```python
from build123d import *

# Parameters (mm, degrees)
SKETCH_1_R          = 1.65
EXTRUDE_1_DEPTH     = 20
CUT_EXTRUDE_START   = -15
SKETCH_4_R          = 1.65
CUT_EXTRUDE_1_DEPTH = 15
FILLET_1_R          = 10
FILLET_2_R          = 5


with BuildPart() as part:
    # ｽｹｯﾁ1 → ﾎﾞｽ - 押し出し1 (new body)
    with BuildSketch(Plane(origin=(0, 0, 0), x_dir=(1, 0, 0), z_dir=(0, 1, 0))):
        with BuildLine():
            Line((20.396078054, 5), (20.396078054, -5))
            ThreePointArc((20.396078054, -5), (19.876430019, -6.776985295), (19.202290705, -8.501295883))
            ThreePointArc((19.202290705, -8.501295883), (18.958497792, -12.709351685), (21.542725681, -16.039356915))
            ThreePointArc((21.542725681, -16.039356915), (22.273863607, -22.273863607), (16.039356915, -21.542725681))
            ThreePointArc((16.039356915, -21.542725681), (12.709351685, -18.958497792), (8.501295883, -19.202290705))
            ThreePointArc((8.501295883, -19.202290705), (6.776985295, -19.876430019), (5, -20.396078054))
            Line((5, -20.396078054), (-5, -20.396078054))
            ThreePointArc((-5, -20.396078054), (-6.776985295, -19.876430019), (-8.501295883, -19.202290705))
            ThreePointArc((-8.501295883, -19.202290705), (-12.709351685, -18.958497792), (-16.039356915, -21.542725681))
            ThreePointArc((-16.039356915, -21.542725681), (-22.273863607, -22.273863607), (-21.542725681, -16.039356915))
            ThreePointArc((-21.542725681, -16.039356915), (-18.958497792, -12.709351685), (-19.202290705, -8.501295883))
            ThreePointArc((-19.202290705, -8.501295883), (-19.876430019, -6.776985295), (-20.396078054, -5))
            Line((-20.396078054, -5), (-20.396078054, 5))
            ThreePointArc((-20.396078054, 5), (-19.876430019, 6.776985295), (-19.202290705, 8.501295883))
            ThreePointArc((-19.202290705, 8.501295883), (-18.958497792, 12.709351685), (-21.542725681, 16.039356915))
            ThreePointArc((-21.542725681, 16.039356915), (-22.273863607, 22.273863607), (-16.039356915, 21.542725681))
            ThreePointArc((-16.039356915, 21.542725681), (-12.709351685, 18.958497792), (-8.501295883, 19.202290705))
            ThreePointArc((-8.501295883, 19.202290705), (-6.776985295, 19.876430019), (-5, 20.396078054))
            Line((-5, 20.396078054), (5, 20.396078054))
            ThreePointArc((5, 20.396078054), (6.776985295, 19.876430019), (8.501295883, 19.202290705))
            ThreePointArc((8.501295883, 19.202290705), (12.709351685, 18.958497792), (16.039356915, 21.542725681))
            ThreePointArc((16.039356915, 21.542725681), (22.273863607, 22.273863607), (21.542725681, 16.039356915))
            ThreePointArc((21.542725681, 16.039356915), (18.958497792, 12.709351685), (19.202290705, 8.501295883))
            ThreePointArc((19.202290705, 8.501295883), (19.876430019, 6.776985295), (20.396078054, 5))
        make_face()
        with Locations(Location((19.445436483, 19.445436483, 0), (0, 0, 270))):
            Circle(SKETCH_1_R, mode=Mode.SUBTRACT)
        with Locations(Location((19.445436483, -19.445436483, 0), (0, 0, 270))):
            Circle(SKETCH_1_R, mode=Mode.SUBTRACT)
        with Locations(Location((-19.445436483, -19.445436483, 0), (0, 0, 270))):
            Circle(SKETCH_1_R, mode=Mode.SUBTRACT)
        with Locations(Location((-19.445436483, 19.445436483, 0), (0, 0, 270))):
            Circle(SKETCH_1_R, mode=Mode.SUBTRACT)
        with BuildLine():
            ThreePointArc((10.911844504, 15.554152164), (0, 19), (-10.911844504, 15.554152164))
            ThreePointArc((-10.911844504, 15.554152164), (-14.849242405, 14.849242405), (-15.554152164, 10.911844504))
            ThreePointArc((-15.554152164, 10.911844504), (-19, 0), (-15.554152164, -10.911844504))
            ThreePointArc((-15.554152164, -10.911844504), (-14.849242405, -14.849242405), (-10.911844504, -15.554152164))
            ThreePointArc((-10.911844504, -15.554152164), (0, -19), (10.911844504, -15.554152164))
            ThreePointArc((10.911844504, -15.554152164), (14.849242405, -14.849242405), (15.554152164, -10.911844504))
            ThreePointArc((15.554152164, -10.911844504), (19, 0), (15.554152164, 10.911844504))
            ThreePointArc((15.554152164, 10.911844504), (14.849242405, 14.849242405), (10.911844504, 15.554152164))
        make_face(mode=Mode.SUBTRACT)
    extrude(amount=EXTRUDE_1_DEPTH)

    # ｽｹｯﾁ4 → ｶｯﾄ - 押し出し1 (cut)
    # profile 1 of 3: a face of its own
    with BuildSketch(Plane(origin=(0, 20, 0), x_dir=(1, 0, 0), z_dir=(0, 1, 0)).offset(CUT_EXTRUDE_START)):
        with BuildLine():
            ThreePointArc((-21.542725681, 16.039356915), (-20.338354704, 15.06240992), (-19.424600386, 13.80941833))
            Line((-19.424600386, 13.80941833), (-16.617009355, 16.617009361))
            ThreePointArc((-16.617009355, 16.617009361), (-18.979538151, 15.472661792), (-21.542725681, 16.039356915))
        make_face()
    # profile 2 of 3: a face of its own
    with BuildSketch(Plane(origin=(0, 20, 0), x_dir=(1, 0, 0), z_dir=(0, 1, 0)).offset(CUT_EXTRUDE_START)):
        with BuildLine():
            ThreePointArc((-21.542725681, 16.039356915), (-18.979538151, 15.472661792), (-16.617009355, 16.617009361))
            ThreePointArc((-16.617009355, 16.617009361), (-15.749918352, 17.914702755), (-15.445436483, 19.445436483))
            ThreePointArc((-15.445436483, 19.445436483), (-15.596779686, 20.535317607), (-16.039356915, 21.542725681))
            ThreePointArc((-16.039356915, 21.542725681), (-22.273863607, 22.273863607), (-21.542725681, 16.039356915))
        make_face()
        with Locations(Location((-19.445436483, 19.445436483, 0), (0, 0, 270))):
            Circle(SKETCH_4_R, mode=Mode.SUBTRACT)
    # profile 3 of 3: a face of its own
    with BuildSketch(Plane(origin=(0, 20, 0), x_dir=(1, 0, 0), z_dir=(0, 1, 0)).offset(CUT_EXTRUDE_START)):
        with BuildLine():
            ThreePointArc((-15.445436483, 19.445436483), (-15.749918352, 17.914702755), (-16.617009355, 16.617009361))
            Line((-16.617009355, 16.617009361), (-13.80941833, 19.424600386))
            ThreePointArc((-13.80941833, 19.424600386), (-15.06240992, 20.338354704), (-16.039356915, 21.542725681))
            ThreePointArc((-16.039356915, 21.542725681), (-15.596779686, 20.535317607), (-15.445436483, 19.445436483))
        make_face()
    extrude(amount=CUT_EXTRUDE_1_DEPTH, mode=Mode.SUBTRACT)

    # ﾌｨﾚｯﾄ1
    fillet_1_edges = [part.edges().sort_by_distance(p)[0] for p in [
        (20.396078054, 10, -5),
        (20.396078054, 10, 5),
        (5, 10, 20.396078054),
        (-5, 10, 20.396078054),
        (-20.396078054, 10, 5),
        (-20.396078054, 10, -5),
        (-5, 10, -20.396078054),
        (5, 10, -20.396078054),
        (15.554152164, 10, -10.911844504),
        (10.911844504, 10, -15.554152164),
        (-10.911844504, 10, -15.554152164),
        (-15.554152164, 10, -10.911844504),
        (-15.554152164, 10, 10.911844504),
        (-10.911844504, 10, 15.554152164),
        (10.911844504, 10, 15.554152164),
        (15.554152164, 10, 10.911844504),
    ]]
    fillet(fillet_1_edges, radius=FILLET_1_R)

    # ﾌｨﾚｯﾄ2
    fillet_2_edges = [part.edges().sort_by_distance(p)[0] for p in [
        (-13.80941833, 12.5, -19.424600386),
        (-19.424600386, 12.5, -13.80941833),
    ]]
    fillet(fillet_2_edges, radius=FILLET_2_R)


solid = part.part
```
CAD build for the part. Positions are in the model's coordinates, mm. A direction names the side the tool comes from. Round coordinates to 2 decimals unless told otherwise and drop trailing zeros. Write each loop counter-clockwise with the first axis right and the second up, starting at its lowest first coordinate (ties: lowest second). Pieces come first, ordered by that corner, then holes.
Item 1: Drop flat-ended pins along their axis: pin 1 Ø3.5 at (y, z) = (11.5, -0.5) entering from +X; pin 2 Ø2 at (x, y) = (3.5, 9) entering from +Z; pin 3 Ø6 at (y, z) = (7.5, 0.5) entering from -X. Give the stop position or say it passes through.
Filled in:
pin 1: stops at x = 20.4
pin 2: stops at z = 20.4
pin 3: stops at x = -20.4
Item 2: Band-saw the part on C-C on y = 2.75. Give the number of separate pieces and of enclosed holes in the cut face, then the cut area to 3 significant figures.
Filled in:
separate pieces: 1
enclosed holes: 5
area: 484 mm2
Item 3: Mould opens along Z. For faces 1 (the cylindrical face through (-5.274, 10.14, 20.254)), 2 (the cylindrical face through (-14.9, 9.9, 14.8)), 3 (the cylindrical face through (7.677, 9.86, -19.546)) say: released by +Z, released by -Z, zero draft, split by the parting line, or undercut.
Filled in:
face 1: released by +Z
face 2: undercut
face 3: released by -Z
Item 4: Band-saw the part on B-B on z = 14.5. Write the cut outline in (x, y), then the cut area to 3 significant figures.
Filled in:
outline: (-19.87, 0) - (-15.15, 0) - (-15.15, 20) - (-19.87, 20) - close; (15.15, 0) - (19.87, 0) - (19.87, 20) - (15.15, 20) - close
area: 188 mm2
Item 5: Drill centre lines: L1, parallel to X at y = 11, z = 20.5; L2, parallel to X at y = 4.75, z = -17; L3, parallel to Z at x = 12, y = 9. Where is each one in solid material? Low to high.
Filled in:
L1: x = -23.3 to -20.71, -18.18 to -15.23, 15.23 to 18.18, 20.71 to 23.3
L2: x = -22.61 to -8.49, 8.49 to 22.61
L3: z = -18.78 to -15.92, 15.92 to 18.78
Item 6: Tool access for faces 4 (the flat face through (20.396, 10, 0)), 5 (the cylindrical face through (-14.8, 9.9, -14.9)), 6 (the flat face through (0, 10, 20.396)): list every direction of +Z, -Z, +X, -X, +Y, -Y with a clear straight run to the whole face (end or side of a thin tool).
Filled in:
face 4: +X, +Y, -Y
face 5: +Y, -Y
face 6: +Z, +Y, -Y
Item 7: Band-saw the part on A-A on x = 0. Write the cut outline in (y, z).
Filled in:
outline: (0, -20.4) - (20, -20.4) - (20, -19) - (0, -19) - close; (0, 19) - (20, 19) - (20, 20.4) - (0, 20.4) - close
